The figure shows three views and two pictorial views of one solid part (mm, origin at its lowest corner). Answer the questions. A direction names the side the tool comes from. Give positions to 0.01 mm unless a question says otherwise; leave off trailing zeros. Order: outer loops, then holes, each group sorted by start corner. A loop starts at its lowest first (then second) coordinate and runs counter-clockwise, first axis right, second up. Notation, with made-up numbers: (21.5, -15) -> (30.5, -15) arc R20 ccw to (30.5, 16) -> close; hole circle Ø1 at (-32, 43). An arc over 180 degrees is marked (long way). Use one line per item in the form item = value.
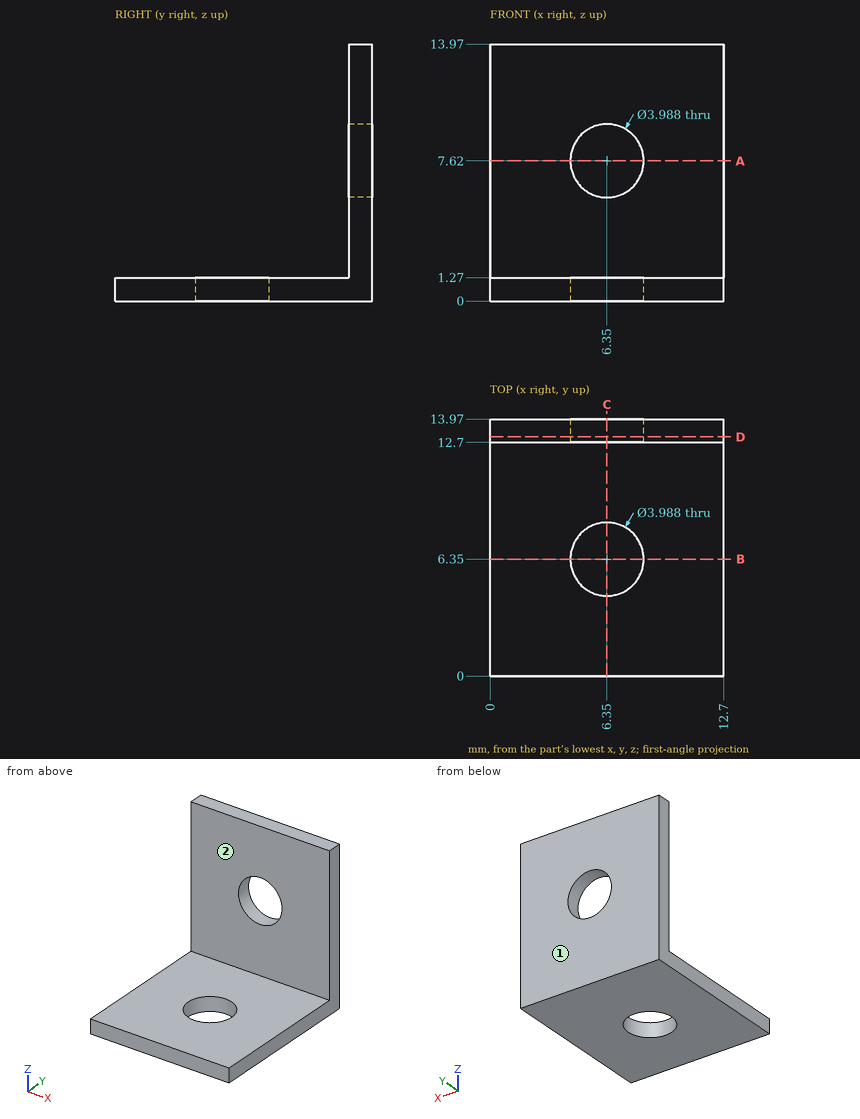
Item 1: The part is cut by section C-C on x = 6.35. Give the vertices of the cut face in (y, z).
Checks:
outline = (0, 0) -> (4.36, 0) -> (4.36, 1.27) -> (0, 1.27) -> close; (8.34, 0) -> (13.97, 0) -> (13.97, 5.63) -> (12.7, 5.63) -> (12.7, 1.27) -> (8.34, 1.27) -> close; (12.7, 9.61) -> (13.97, 9.61) -> (13.97, 13.97) -> (12.7, 13.97) -> close
Item 2: Given pin 1 Ø3.5 at (x, y) = (6.35, 6.35) entering from +Z; pin 2 Ø6.5 at (x, y) = (9.5, 8) entering from +Z; pin 3 Ø4 at (x, z) = (4.5, 10.5) entering from -Y, each flat-ended and moving along its own axis, determine where each tip first touches the part or whether it passes through.
Checks:
pin_1 = through
pin_2 = 1.27
pin_3 = 12.7
Item 3: Straight lines are drawn through the part: L1, parallel to Y at x = 6.35, z = 0.55; L2, parallel to Z at x = 6.35, y = 13.25; L3, parallel to Z at x = 2.25, y = 9.75. For each, find the intervals that lie inside material, in ascending order. Write a range as from..to.
Checks:
L1 = 0..4.36, 8.34..13.97
L2 = 0..5.63, 9.61..13.97
L3 = 0..1.27
Item 4: The part is cut by section B-B on y = 6.35. Give the vertices of the cut face in (x, z), and give its area (3 significant figures).
Checks:
outline = (0, 0) -> (4.36, 0) -> (4.36, 1.27) -> (0, 1.27) -> close; (8.34, 0) -> (12.7, 0) -> (12.7, 1.27) -> (8.34, 1.27) -> close
area = 11.1 mm²
Item 5: Which of the six approach directions +Z, -Z, +X, -X, +Y, -Y give full straight-line access (tool end or side, diameter ignored) to the marked faces 1 and 2?
Checks:
face_1 = +Z, -Z, +X, -X, +Y
face_2 = +Z, +X, -X, -Y
Item 6: The part is cut by section D-D on y = 13. Give the vertices of the cut face in (x, z).
Checks:
outline = (0, 0) -> (12.7, 0) -> (12.7, 13.97) -> (0, 13.97) -> close; hole circle Ø3.99 at (6.35, 7.62)
Item 7: The part is cut by section A-A on z = 7.62. Give the vertices of the cut face in (x, y), and give its area (3 significant figures).
Checks:
outline = (0, 12.7) -> (4.36, 12.7) -> (4.36, 13.97) -> (0, 13.97) -> close; (8.34, 12.7) -> (12.7, 12.7) -> (12.7, 13.97) -> (8.34, 13.97) -> close
area = 11.1 mm²
